Build history of the part. All positions in model axes, mm. Face numbers are marked on the shaded views. A direction names the side the tool comes from. Round coordinates to 2 decimals unless told otherwise and drop trailing zeros. Write each loop counter-clockwise with the first axis right and the second up, starting at its lowest first coordinate (ties: lowest second). Pieces come first, ordered by that corner, then holes. Notation, with made-up numbers: (-12.5, 54) -> (42.5, 54) arc R16 ccw to (42.5, 82) -> close; hole circle Ø10 at (-15, 33.5). An arc over 180 degrees is marked (long way). Answer as CSV lines item,"result".
from build123d import *

# Parameters (mm, degrees)
F0_W     = 152.4
F0_H     = 63.5
F1_DEPTH = 304.8
F2_R     = 5.08
F3_R     = 38.1
F4_DEPTH = 254


with BuildPart() as f1:
    # F0 (on Front) → F1 (new body)
    with BuildSketch(Plane.XZ):
        Rectangle(F0_W, F0_H)
    extrude(amount=F1_DEPTH)

    # F2
    f2_edges = [f1.edges().sort_by_distance(p)[0] for p in [
        (76.2, -152.4, 31.75),
        (76.2, -304.8, 0),
        (76.2, 0, 0),
        (0, 0, 31.75),
        (-76.2, 0, 0),
        (-76.2, -152.4, 31.75),
        (-76.2, -304.8, 0),
        (0, -304.8, 31.75),
    ]]
    fillet(f2_edges, radius=F2_R)

    # F3 (on Front) → F4 (join)
    with BuildSketch(Plane.XZ):
        with Locations((0, 26.523461)):
            Circle(F3_R)
    extrude(amount=F4_DEPTH)


solid = f1.part
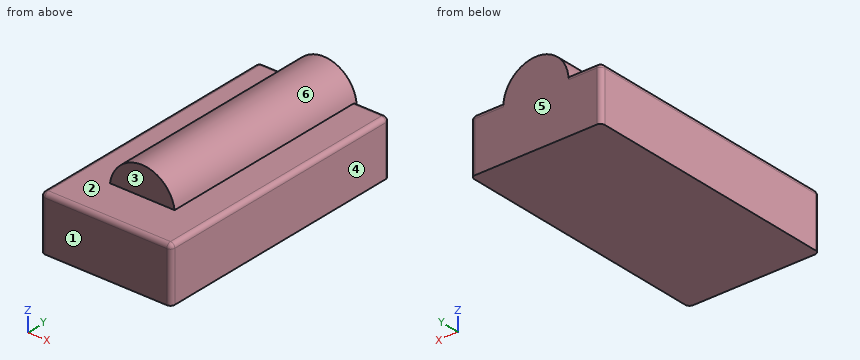
1. Which spindle directions (+Z, -Z, +X, -X, +Y, -Y) get a long thin tool onto all of the face, cutting with end or side? Do the marked faces 1, 2 and 3. Say none if no direction does.
Results found:
face 1,"+Z, -Z, +X, -X, -Y"
face 2,"+Z, -Y"
face 3,"+Z, +X, -X, -Y"
2. Probe line 1 along Z through (x, y) = (51.5, -99.5); line 2 along Y through (x, z) = (12, 46.5); line 3 along Z through (x, y) = (-1, -115). List the from-to ranges inside material, lowest first.
Results found:
line 1,"z = -31.75 to 31.75"
line 2,"y = -254 to 0"
line 3,"z = -31.75 to 64.61"
3. Drop a flat-ended pin along its axis: pin 1 Ø1 at (x, z) = (23, 46) entering from -Y. Give the stop position or say it passes through.
Results found:
pin 1,"stops at y = -254"
4. Cut at B-B, the plane y = -127. Write the cut outline in (x, z).
Results found:
outline,"(-76.2, -31.75) -> (76.2, -31.75) -> (76.2, 26.67) arc R5.08 ccw to (71.12, 31.75) -> (37.74, 31.75) arc R38.1 ccw to (-37.74, 31.75) -> (-71.12, 31.75) arc R5.08 ccw to (-76.2, 26.67) -> close"
5. Mould opens along X. For the marked faces 4, 5 and 6 say: +X half, -X half, draft (parallel to the pull), parting line (faces both ways), or undercut.
Results found:
face 4,"+X half"
face 5,"draft"
face 6,"parting line"
6. Cut at A-A, the plane x = 0. Write the cut outline in (y, z).
Results found:
outline,"(-304.8, -31.75) -> (0, -31.75) -> (0, 64.62) -> (-254, 64.62) -> (-254, 31.75) -> (-299.72, 31.75) arc R5.08 ccw to (-304.8, 26.67) -> close"
7. Cut at C-C, the plane x = 67.5. Write the cut outline in (y, z).
Results found:
outline,"(-304.8, -31.75) -> (0, -31.75) -> (0, 26.67) arc R5.08 ccw to (-5.08, 31.75) -> (-299.72, 31.75) arc R5.08 ccw to (-304.8, 26.67) -> close"
